from build123d import *

# Parameters (mm, degrees)
SKETCH_1_W          = 40
SKETCH_1_H          = 12
SKETCH_1_R          = 3.6
EXTRUDE_1_DEPTH     = 15
SKETCH_2_R          = 2.5
CUT_EXTRUDE_1_DEPTH = 13


with BuildPart() as part:
    # Эскиз1 → Бобышка-Вытянуть1 (new body)
    with BuildSketch(Plane(origin=(0, 0, 0), x_dir=(1, 0, 0), z_dir=(0, 1, 0))):
        Rectangle(SKETCH_1_W, SKETCH_1_H)
        Circle(SKETCH_1_R, mode=Mode.SUBTRACT)
    extrude(amount=EXTRUDE_1_DEPTH)

    # Эскиз2 → Вырез-Вытянуть1 (cut, through all)
    with BuildSketch(Plane.XY.offset(6)):
        with Locations((-15, 7.5)):
            Circle(SKETCH_2_R)
        with Locations((15, 7.5)):
            Circle(SKETCH_2_R)
    extrude(amount=-CUT_EXTRUDE_1_DEPTH, mode=Mode.SUBTRACT)


solid = part.part
The model under review builds one solid part; all positions refer to its coordinate system, in mm. Give positions to 0.01 mm unless a question says otherwise; leave off trailing zeros. Write each loop counter-clockwise with the first axis right and the second up, starting at its lowest first coordinate (ties: lowest second). Pieces come first, ordered by that corner, then holes.
1. Wall thickness on L1, parallel to Y at x = 15, z = -3; L2, parallel to X at y = 6, z = 0; L3, parallel to X at y = 10.5, z = 1.5: over which ranges is each line inside the solid? List them lowest first.
2. Draft analysis for pull direction X (two halves, no side actions). For faces 1 (the flat face through (-20, 7, 0)), 2 (the flat face through (0, 7, 6)), 3 (the cylindrical face through (-17, 6, 0)), state which applies: +X half, -X half, draft (parallel to the pull), parting line (faces both ways), or undercut.
3. For P1, Ø4.5, axis at x = 15, y = 7.5, coming from the +Z side, flat-tipped, find the tip position at first contact; note if it passes through.
4. Add section D-D, the plane y = 2.75. Write out the cut boundary in (x, z).
5. Add section C-C, the plane x = 0. Write out the cut boundary in (y, z).
6. Add section B-B, the plane y = 7.5. Write out the cut boundary in (x, z), plus the area to 3 significant figures.
7. Add section A-A, the plane z = 0. Write out the cut boundary in (x, y), plus the area to 3 significant figures.
Worked answers:
1. L1: y = 0 to 5, 10 to 15
1. L2: x = -20 to -17, -13 to -3.6, 3.6 to 13, 17 to 20
1. L3: x = -20 to -3.27, 3.27 to 20
2. face 1: -X half
2. face 2: draft
2. face 3: undercut
3. P1: passes through
4. outline: (-20, -6) - (20, -6) - (20, 6) - (-20, 6) - close; hole circle Ø7.2 at (0, 0)
5. outline: (0, -6) - (15, -6) - (15, -3.6) - (0, -3.6) - close; (0, 3.6) - (15, 3.6) - (15, 6) - (0, 6) - close
6. outline: (-20, -6) - (-17.5, -6) - (-17.5, 6) - (-20, 6) - close; (-12.5, -6) - (12.5, -6) - (12.5, 6) - (-12.5, 6) - close; (17.5, -6) - (20, -6) - (20, 6) - (17.5, 6) - close; hole circle Ø7.2 at (0, 0)
6. area: 319 mm2
7. outline: (-20, 0) - (-3.6, 0) - (-3.6, 15) - (-20, 15) - close; (3.6, 0) - (20, 0) - (20, 15) - (3.6, 15) - close; hole circle Ø5 at (-15, 7.5); hole circle Ø5 at (15, 7.5)
7. area: 453 mm2
